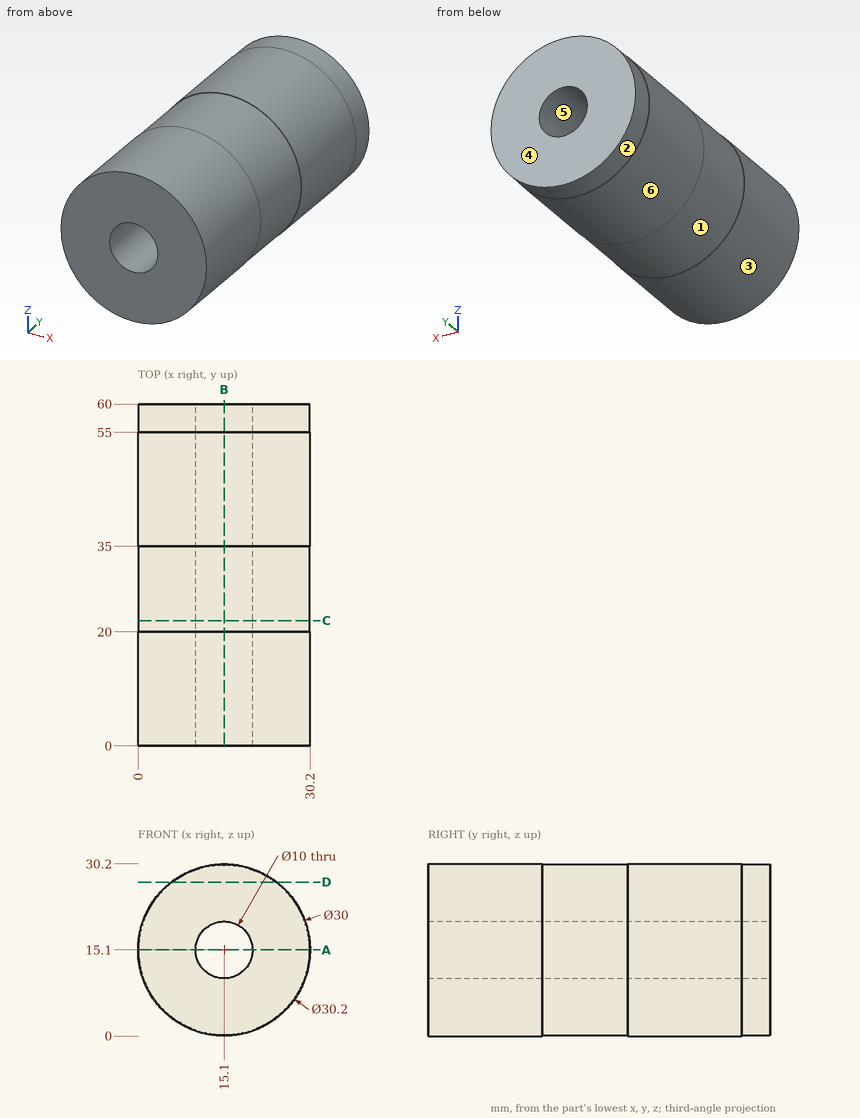
Could you check a few things on this drawing? It's one solid part, dimensions in mm from its lowest x, y, z. A direction names the side the tool comes from. Give positions to 0.01 mm unless a question says otherwise; leave off trailing zeros. Order: outer loops, then holes, each group sorted by start corner. A loop starts at its lowest first (then second) coordinate and runs counter-clockwise, first axis right, second up.
1. Suppose I cut it at A-A (z = 15.1). Write out the boundary of the cut face in (x, y).
Answers below:
outline: (0, 0) - (10.1, 0) - (10.1, 60) - (0.1, 60) - (0.1, 55) - (0, 55) - (0, 35) - (0.1, 35) - (0.1, 20) - (0, 20) - close; (20.1, 0) - (30.2, 0) - (30.2, 20) - (30.1, 20) - (30.1, 35) - (30.2, 35) - (30.2, 55) - (30.1, 55) - (30.1, 60) - (20.1, 60) - close
2. Suppose I cut it at B-B (x = 15.1). Write out the boundary of the cut face in (y, z).
Answers below:
outline: (0, 0) - (20, 0) - (20, 0.1) - (35, 0.1) - (35, 0) - (55, 0) - (55, 0.1) - (60, 0.1) - (60, 10.1) - (0, 10.1) - close; (0, 20.1) - (60, 20.1) - (60, 30.1) - (55, 30.1) - (55, 30.2) - (35, 30.2) - (35, 30.1) - (20, 30.1) - (20, 30.2) - (0, 30.2) - close
3. Thinking about a two-plate mould opening in Z: for the marked faces 4, 5 and 6, which applies, +Z half, -Z half, draft (parallel to the pull), parting line (faces both ways), or undercut?
Answers below:
face 4: draft
face 5: undercut
face 6: parting line
4. Which directions (+Z, -Z, +X, -X, +Y, -Y) give clear straight access to the entire face, cutting with the end or side of a thin tool? Please do the marked faces 1, 2 and 3.
Answers below:
face 1: none
face 2: +Y
face 3: +Y, -Y
5. I need wall thicknesses on L1, parallel to Y at x = 22.5, z = 2; L2, parallel to Z at x = 15, y = 29. Which ranges of each line are inside material? Lowest first, please.
Answers below:
L1: y = 0 to 20, 35 to 55
L2: z = 0.1 to 10.1, 20.1 to 30.1
6. Suppose I cut it at C-C (y = 22). Write out the boundary of the cut face in (x, z), plus the area to 3 significant figures.
Answers below:
outline: circle Ø30 at (15.1, 15.1); hole circle Ø10 at (15.1, 15.1)
area: 628 mm2
7. Suppose I cut it at D-D (z = 27). Write out the boundary of the cut face in (x, y), plus the area to 3 significant figures.
Answers below:
outline: (5.8, 0) - (24.4, 0) - (24.4, 20) - (24.23, 20) - (24.23, 35) - (24.4, 35) - (24.4, 55) - (24.23, 55) - (24.23, 60) - (5.97, 60) - (5.97, 55) - (5.8, 55) - (5.8, 35) - (5.97, 35) - (5.97, 20) - (5.8, 20) - close
area: 1,110 mm2
8. For pin 1 (8 mm diameter, centred on x = 15.1, z = 15.1, fed in from -Y); pin 2 (8 mm diameter, centred on y = 9, z = 25, fed in from -X); pin 3 (10 mm diameter, centred on x = 24.5, y = 50, fed in from +Z); pin 4 (4 mm diameter, centred on x = 15, y = 28, fed in from -Z), each with a flat end and sliding along its axis, tell me the tip position at first contact or that it passes through.
Answers below:
pin 1: passes through
pin 2: stops at x = 1.2
pin 3: stops at z = 29.54
pin 4: stops at z = 0.1
